Could you check a few things on this model? Use its own coordinates, in mm. Face numbers are marked on the shaded views. A direction names the side the tool comes from. Give positions to 0.01 mm unless a question says otherwise; leave off trailing zeros. Order: outer loops, then holes, each group sorted by start corner. A loop starts at its lowest first (then second) coordinate and runs counter-clockwise, first axis right, second up.
Autodesk Inventor part; units mm, degrees
ref_plane "YZ Plane" through (0, 0, 0) normal (1, 0, 0) x (0, 1, 0)
ref_plane "XZ Plane" through (0, 0, 0) normal (0, 1, 0) x (-1, 0, 0)
ref_plane "XY Plane" through (0, 0, 0) normal (0, 0, 1) x (1, 0, 0)
sketch "Skizze1" plane through (0, 0, 0) normal (0, 0, 1) x (1, 0, 0)
  line L0 (40, 37) -> (56, 37)
  line L1 (56, 37) -> (56, -25)
  line L2 (40, -9) -> (40, 37)
  line L3 (56, -25) -> (0, -25)
  line L4 (40, -9) -> (23.3238, -9)
  line L5 (0, 25) -> (-64, 25)
  line L6 (-64, 25) -> (-64, 9)
  line L7 (-64, 9) -> (-23.3238, 9)
  arc A0 (23.3238, -9) -> (0, 25) centre (0, 0) ccw
  arc A1 (-23.3238, 9) -> (0, -25) centre (0, 0) ccw
  dimension "d0" = 16
  dimension "d1" = 25
  dimension "d2" = 62
  dimension "d3" = 56
  dimension "d4" = 16
  dimension "d5" = 120
  dimension "d6" = 16
  dimension "d7" = 25
extrude "Extrusion1" add sketch "Skizze1" along normal blind 75
sketch "Skizze2" plane through (0, 0, 75) normal (0, 0, 1) x (1, 0, 0)
  circle A0 centre (0, 0) radius 12.5
  dimension "d10" = 25
extrude "Extrusion2" cut sketch "Skizze2" against normal up to surface (75 mm away)
chamfer "Fasen1" distance 13 angle 45 2 edges at (48, 37, 75) (48, 37, 0)
sketch "Skizze3" plane through (56, -25, 75) normal (1, 0, 0) x (0, 0, -1)
  line L0 (62, 62) -> (13, 62)
  point P0 (75, 25)
  point P1 (37.5, 42)
  point P2 (37.5, 62)
  dimension "d23" = 20
hole "Bohrung1" at (56, 17, 37.5) direction (-1, 0, 0) diameter 20 depth 16
sketch "Skizze4" plane through (-64, 25, 0) normal (0, 1, 0) x (1, 0, 0)
  line L0 (0, 0) -> (0, -75)
  line L1 (0, -37.5) -> (64, -37.5) construction
  line L2 (64, 0) -> (64, -75)
  point P0 (16, -59.5)
  point P1 (16, -15.5)
  dimension "d31" = 44
  dimension "d32" = 16
hole "Bohrung2" at (-48, 25, 59.5) at (-48, 25, 15.5) direction (0, -1, 0) diameter 12 end through all
equation "\"d0\" = d4"
equation "\"d6\" = d0"
properties part number "practice4" material "Stahl, galvanisiert"
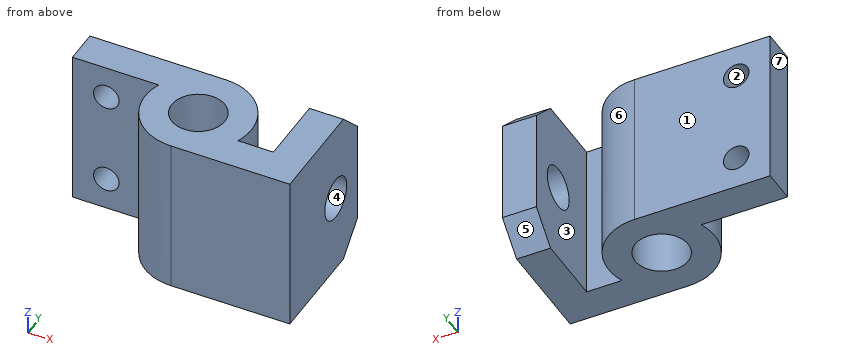
Item 1: For pin 1 (11 mm diameter, centred on x = -48, z = 15.5, fed in from +Y); pin 2 (2 mm diameter, centred on y = -3, z = 30.5, fed in from -X); pin 3 (1 mm diameter, centred on x = -19, z = 42.5, fed in from -Y); pin 4 (8.5 mm diameter, centred on x = 29.5, z = 38.5, fed in from +Y), each with a flat end and sliding along its axis, tell me the tip position at first contact or that it passes through.
Findings:
pin 1: passes through
pin 2: stops at x = -24.92
pin 3: stops at y = -16.82
pin 4: stops at y = -9
Item 2: Please list where these lines run through material, in increasing order: line 1 along Z through (x, y) = (-48, 13.5); line 2 along X through (y, z) = (-0.5, 7.5) (3 decimals); line 3 along Y through (x, z) = (0, 18.5).
Findings:
line 1: z = 0 to 9.5, 21.5 to 53.5, 65.5 to 75
line 2: x = -24.995 to -12.49, 12.49 to 24.995, 40 to 56
line 3: y = -25 to -12.5, 12.5 to 25
Item 3: Imagine slicing it at A-A on z = 37.5. List the corners of the cut face in (x, y) for me.
Findings:
outline: (-64, 9) - (-23.32, 9) arc R25 ccw to (0, -25) - (56, -25) - (56, 7) - (40, 7) - (40, -9) - (23.32, -9) arc R25 ccw to (0, 25) - (-64, 25) - close; (40, 27) - (56, 27) - (56, 37) - (40, 37) - close; hole circle Ø25 at (0, 0)
Item 4: Imagine slicing it at D-D on y = 0. List the corners of the cut face in (x, z) for me.
Findings:
outline: (-25, 0) - (-12.5, 0) - (-12.5, 75) - (-25, 75) - close; (12.5, 0) - (25, 0) - (25, 75) - (12.5, 75) - close; (40, 0) - (56, 0) - (56, 75) - (40, 75) - close
Item 5: Imagine slicing it at C-C on y = 17. List the corners of the cut face in (x, z) for me, then the cut area to 3 significant figures.
Findings:
outline: (-64, 0) - (18.33, 0) - (18.33, 75) - (-64, 75) - close; (40, 0) - (56, 0) - (56, 27.5) - (40, 27.5) - close; (40, 47.5) - (56, 47.5) - (56, 75) - (40, 75) - close; hole circle Ø12 at (-48, 15.5); hole circle Ø12 at (-48, 59.5)
area: 6,830 mm2
Item 6: Imagine slicing it at B-B on x = -48. List the corners of the cut face in (y, z) for me.
Findings:
outline: (9, 0) - (25, 0) - (25, 9.5) - (9, 9.5) - close; (9, 21.5) - (25, 21.5) - (25, 53.5) - (9, 53.5) - close; (9, 65.5) - (25, 65.5) - (25, 75) - (9, 75) - close
Item 7: We'd pull the mould along Y, two halves only. Please class the marked faces 5, 6 and 7: +Y half, -Y half, draft (parallel to the pull), parting line (faces both ways), or undercut.
Findings:
face 5: +Y half
face 6: undercut
face 7: draft
Item 8: For the marked faces 1, 2, 3 and 4, which set-ups out of +Z, -Z, +X, -X, +Y, -Y let a thin tool reach every point of the face, with its end or its side?
Findings:
face 1: +Z, -Z, -X, +Y
face 2: +Y, -Y
face 3: +Z, -Z, +Y
face 4: +X
